Verification items for the finished model (mm, model axes). A direction names the side the tool comes from. Give positions to 0.01 mm unless a question says otherwise; leave off trailing zeros. Write each loop counter-clockwise with the first axis right and the second up, starting at its lowest first coordinate (ties: lowest second). Pieces come first, ordered by that corner, then holes. Notation, with made-up numbers: M 51.5,-20 L 103.5,-20 A13 ccw 103.5,5 Z; hole C -19,27 d7. An arc over 180 degrees is marked long. Answer as a JSON object with one key per item and string values.
```python
from build123d import *

# Parameters (mm, degrees)
ESQUISSE2_R        = 1.95
BOSS_EXTRU_1_DEPTH = 10
CONG_1_R           = 10
BOSS_EXTRU_2_DEPTH = 10
ESQUISSE4_R        = 1.95
BOSS_EXTRU_3_DEPTH = 10


with BuildPart() as part:
    # Esquisse2 → Boss.-Extru.1 (new body)
    # profile 1 of 3: a face of its own
    with BuildSketch(Plane(origin=(0, 0, 0), x_dir=(1, 0, 0), z_dir=(0, 1, 0))):
        with BuildLine():
            Line((-5, 90), (-5, 0))
            ThreePointArc((-5, 0), (0, -5), (5, 0))
            Line((5, 0), (5, 87.928932188))
            Line((5, 87.928932188), (3.535533906, 86.464466094))
            ThreePointArc((3.535533906, 86.464466094), (-1.913417162, 85.380602337), (-5, 90))
        make_face()
    # profile 2 of 3: a face of its own
    with BuildSketch(Plane(origin=(0, 0, 0), x_dir=(1, 0, 0), z_dir=(0, 1, 0))):
        with BuildLine():
            Line((38.890872965, 135.961940777), (-3.535533906, 93.535533906))
            ThreePointArc((-3.535533906, 93.535533906), (1.913417162, 94.619397663), (5, 90))
            Line((5, 90), (5, 87.928932188))
            Line((5, 87.928932188), (45.961940777, 128.890872965))
            ThreePointArc((45.961940777, 128.890872965), (45.961940777, 135.961940777), (38.890872965, 135.961940777))
        make_face()
        with Locations(Location((42.426406871, 132.426406871, 0), (0, 0, 270))):
            Circle(ESQUISSE2_R, mode=Mode.SUBTRACT)
    # profile 3 of 3: a face of its own
    with BuildSketch(Plane(origin=(0, 0, 0), x_dir=(1, 0, 0), z_dir=(0, 1, 0))):
        with BuildLine():
            ThreePointArc((-3.535533906, 93.535533906), (-4.619397663, 91.913417162), (-5, 90))
            ThreePointArc((-5, 90), (-1.913417162, 85.380602337), (3.535533906, 86.464466094))
            Line((3.535533906, 86.464466094), (5, 87.928932188))
            Line((5, 87.928932188), (5, 90))
            ThreePointArc((5, 90), (1.913417162, 94.619397663), (-3.535533906, 93.535533906))
        make_face()
        with Locations(Location((0, 90, 0), (0, 0, 270))):
            Circle(ESQUISSE2_R, mode=Mode.SUBTRACT)
    extrude(amount=BOSS_EXTRU_1_DEPTH)

    # Congé1
    cong_1_edges = [part.edges().sort_by_distance(p)[0] for p in [
        (5, 5, -87.928932188),
    ]]
    fillet(cong_1_edges, radius=CONG_1_R)

    # Esquisse3 → Boss.-Extru.2 (add)
    with BuildSketch(Plane(origin=(0, 10, 0), x_dir=(1, 0, 0), z_dir=(0, 1, 0))):
        with BuildLine():
            Line((-5, 0), (-5, 70))
            ThreePointArc((-5, 70), (0, 75), (5, 70))
            Line((5, 70), (5, 0))
            ThreePointArc((5, 0), (0, -5), (-5, 0))
        make_face()
        with BuildLine():
            Line((31.819805153, 114.748737342), (17.67766953, 100.606601718))
            ThreePointArc((17.67766953, 100.606601718), (10.606601718, 100.606601718), (10.606601718, 107.67766953))
            Line((10.606601718, 107.67766953), (24.748737342, 121.819805153))
            ThreePointArc((24.748737342, 121.819805153), (31.819805153, 121.819805153), (31.819805153, 114.748737342))
        make_face()
    extrude(amount=BOSS_EXTRU_2_DEPTH)

    # Esquisse4 → Boss.-Extru.3 (add)
    # profile 1 of 4: a face of its own
    with BuildSketch(Plane(origin=(0, 20, 0), x_dir=(1, 0, 0), z_dir=(0, 1, 0))):
        with BuildLine():
            Line((31.819805153, 114.748737342), (45.961940777, 128.890872965))
            ThreePointArc((45.961940777, 128.890872965), (45.961940777, 135.961940777), (38.890872965, 135.961940777))
            Line((38.890872965, 135.961940777), (24.748737342, 121.819805153))
            ThreePointArc((24.748737342, 121.819805153), (31.819805153, 121.819805153), (31.819805153, 114.748737342))
        make_face()
        with Locations(Location((42.426406871, 132.426406871, 0), (0, 0, 270))):
            Circle(ESQUISSE4_R, mode=Mode.SUBTRACT)
    # profile 2 of 4: a face of its own
    with BuildSketch(Plane(origin=(0, 20, 0), x_dir=(1, 0, 0), z_dir=(0, 1, 0))):
        with BuildLine():
            Line((17.67766953, 100.606601718), (31.819805153, 114.748737342))
            ThreePointArc((31.819805153, 114.748737342), (31.819805153, 121.819805153), (24.748737342, 121.819805153))
            Line((24.748737342, 121.819805153), (10.606601718, 107.67766953))
            ThreePointArc((10.606601718, 107.67766953), (10.606601718, 100.606601718), (17.67766953, 100.606601718))
        make_face()
    # profile 3 of 4: a face of its own
    with BuildSketch(Plane(origin=(0, 20, 0), x_dir=(1, 0, 0), z_dir=(0, 1, 0))):
        with BuildLine():
            ThreePointArc((7.928932188, 90.857864376), (5.761204675, 87.613630888), (5, 83.786796564))
            Line((5, 83.786796564), (5, 70))
            ThreePointArc((5, 70), (0, 75), (-5, 70))
            Line((-5, 70), (-5, 90))
            ThreePointArc((-5, 90), (-4.619397663, 91.913417162), (-3.535533906, 93.535533906))
            Line((-3.535533906, 93.535533906), (10.606601718, 107.67766953))
            ThreePointArc((10.606601718, 107.67766953), (10.606601718, 100.606601718), (17.67766953, 100.606601718))
            Line((17.67766953, 100.606601718), (7.928932188, 90.857864376))
        make_face()
        with Locations(Location((0, 90, 0), (0, 0, 270))):
            Circle(ESQUISSE4_R, mode=Mode.SUBTRACT)
    # profile 4 of 4: a face of its own
    with BuildSketch(Plane(origin=(0, 20, 0), x_dir=(1, 0, 0), z_dir=(0, 1, 0))):
        with BuildLine():
            Line((-5, 70), (-5, 0))
            ThreePointArc((-5, 0), (0, -5), (5, 0))
            Line((5, 0), (5, 70))
            ThreePointArc((5, 70), (0, 75), (-5, 70))
        make_face()
    extrude(amount=BOSS_EXTRU_3_DEPTH)


solid = part.part
```
1) Section check B-B on y = 23. Record the boundary of the cut face in (x, z).
Completed:
{"outline": "M -5,-90 A5 ccw -3.54,-93.54 L 38.89,-135.96 A5 ccw 45.96,-128.89 L 7.93,-90.86 A10 cw 5,-83.79 L 5,0 A5 ccw -5,0 Z; hole C 0,-90 d3.9; hole C 42.43,-132.43 d3.9"}
2) Release check for a two-part mould opening along Y. For faces 4 (the face through (2, 0, -72)), 5 (the face through (0.086, 24.93, -91.948)), 6 (the face through (39, 20, -128)), 7 (the face through (0, 15, -75)) record: pulls with the +Y half, pulls with the -Y half, needs draft (parallel to the pull), parting line crosses it, or undercut.
Completed:
{"face 4": "pulls with the -Y half", "face 5": "needs draft", "face 6": "undercut", "face 7": "undercut"}
3) Section check D-D on z = -47. Record the boundary of the cut face in (x, y).
Completed:
{"outline": "M -5,0 L 5,0 L 5,30 L -5,30 Z"}
4) Section check A-A on z = -86. Record the boundary of the cut face in (x, y), and give its area (3 significant figures).
Completed:
{"outline": "M -5,0 L 5.25,0 L 5.25,10 L -5,10 Z; M -5,20 L 5.25,20 L 5.25,30 L -5,30 Z", "area": "205 mm2"}
5) Section check C-C on x = 21.5. Record the boundary of the cut face in (y, z), and give its area (3 significant figures).
Completed:
{"outline": "M 0,-118.57 L 30,-118.57 L 30,-104.43 L 0,-104.43 Z", "area": "424 mm2"}
6) Go/stop test with flat-tipped pins: pin 1 (8 mm diameter, centred on x = 18.5, y = 5.5, fed in from -Z); pin 2 (12 mm diameter, centred on x = 10, y = 25.5, fed in from -Z); pin 3 (4 mm diameter, centred on y = 24.5, z = -57.5, fed in from +X); pin 4 (3.5 mm diameter, centred on x = 42.43, z = -132.43, fed in from -Y). Record where each tip stops, or that it passes through.
Completed:
{"pin 1": "stops at z = -119.57", "pin 2": "stops at z = -113.07", "pin 3": "stops at x = 5", "pin 4": "passes through"}
7) Thickness scan on L1, parallel to Y at x = 32, z = -128.5; L2, parallel to X at y = 29.25, z = -53; L3, parallel to X at y = 4.25, z = -90. Record the ranges inside material, lowest first.
Completed:
{"L1": "y = 0 to 10, 20 to 30", "L2": "x = -5 to 5", "L3": "x = -5 to -1.95, 1.95 to 7.16"}
8) Access from +Z, -Z, +X, -X, +Y, -Y to the whole of each face (thin tool, end or side, straight path). Record for faces 1 (the face through (5, 15, -42)), 2 (the face through (31.74, 14.93, -121.9)), 3 (the face through (-5, 15, -44)).
Completed:
{"face 1": "+Z, +X, +Y, -Y", "face 2": "none", "face 3": "+Z, -Z, -X, +Y, -Y"}
